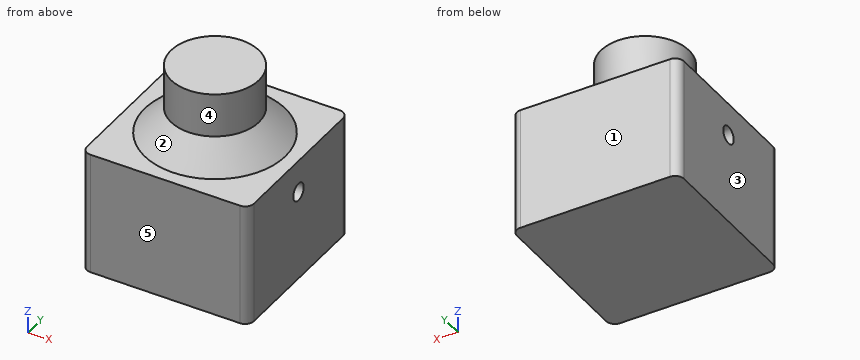
```python
from build123d import *

# Parameters (mm, degrees)
SKETCH1_W           = 19
SKETCH1_H           = 19
BOSS_EXTRUDE1_DEPTH = 14
FILLET1_R           = 1
SKETCH2_R           = 5
BOSS_EXTRUDE2_DEPTH = 8
CHAMFER1_SIZE       = 3
SKETCH3_R           = 1
CUT_EXTRUDE1_DEPTH  = 5
CUT_EXTRUDE2_START  = -5
SKETCH4_R           = 1
CUT_EXTRUDE2_DEPTH  = 5


with BuildPart() as part:
    # Sketch1 → Boss-Extrude1 (new body)
    with BuildSketch(Plane.XY):
        with Locations((66.227433771, 51.961607523)):
            Rectangle(SKETCH1_W, SKETCH1_H)
    extrude(amount=BOSS_EXTRUDE1_DEPTH)

    # Fillet1
    fillet1_edges = [part.edges().sort_by_distance(p)[0] for p in [
        (56.727433771, 61.461607523, 7),
        (75.727433771, 61.461607523, 7),
        (75.727433771, 42.461607523, 7),
        (56.727433771, 42.461607523, 7),
    ]]
    fillet(fillet1_edges, radius=FILLET1_R)

    # Sketch2 → Boss-Extrude2 (add)
    with BuildSketch(Plane.XY.offset(14)):
        with Locations((66.227433771, 51.961607523)):
            Circle(SKETCH2_R)
    extrude(amount=BOSS_EXTRUDE2_DEPTH)

    # Chamfer1
    chamfer1_edges = [part.edges().sort_by_distance(p)[0] for p in [
        (61.227433771, 51.961607523, 14),
    ]]
    chamfer(chamfer1_edges, length=CHAMFER1_SIZE)

    # Sketch3 → Cut-Extrude1 (cut)
    with BuildSketch(Plane.ZY.offset(-56.727433771)):
        with Locations(Location((10.3, 51.961607523, 0), (0, 0, 270))):
            Circle(SKETCH3_R)
    extrude(amount=-CUT_EXTRUDE1_DEPTH, mode=Mode.SUBTRACT)

    # Sketch4 → Cut-Extrude2 (cut)
    with BuildSketch(Plane(origin=(75.727433771, 0, 0), x_dir=(0, 0, -1), z_dir=(1, 0, 0)).offset(CUT_EXTRUDE2_START)):
        with Locations(Location((-10.3, 51.961607523, 0), (0, 0, 270))):
            Circle(SKETCH4_R)
    extrude(amount=CUT_EXTRUDE2_DEPTH, mode=Mode.SUBTRACT)


solid = part.part
```
Here's how the part is built. I have some questions about the finished solid (model axes, mm). Face numbers are marked on the shaded views. A direction names the side the tool comes from. Coordinates: 2 decimals unless noted, no trailing zeros. Loops run counter-clockwise (first coordinate to the right, second up) from the corner with the lowest first, then second, coordinate; pieces in that order, holes last. Notation, with made-up numbers: (-34.75, 71.25) -> (2.25, 71.25) arc R28 ccw to (2.25, 106.25) -> close; hole circle Ø5 at (51.25, 22). An arc over 180 degrees is marked (long way). Return JSON: item names as keys, results as strings.
1) Thinking about a two-plate mould opening in X: for the marked faces 1, 2 and 3, which applies, +X half, -X half, draft (parallel to the pull), parting line (faces both ways), or undercut?
Results below:
{"face 1": "draft", "face 2": "parting line", "face 3": "-X half"}
2) Will these pins go through, and if not, where does the flat tip stop? pin 1 (5 mm diameter, centred on y = 44.5, z = 14.5, fed in from +X); pin 2 (1 mm diameter, centred on y = 52, z = 10, fed in from -X); pin 3 (1.2 mm diameter, centred on y = 51.96, z = 10.3, fed in from +X).
Results below:
{"pin 1": "x = 75.73", "pin 2": "x = 61.73", "pin 3": "x = 70.73"}
3) If we section it at A-A, the plane z = 10.3: Write out the boundary of the cut face in (x, y).
Results below:
{"outline": "(56.73, 43.46) arc R1 ccw to (57.73, 42.46) -> (74.73, 42.46) arc R1 ccw to (75.73, 43.46) -> (75.73, 50.96) -> (70.73, 50.96) -> (70.73, 52.96) -> (75.73, 52.96) -> (75.73, 60.46) arc R1 ccw to (74.73, 61.46) -> (57.73, 61.46) arc R1 ccw to (56.73, 60.46) -> (56.73, 52.96) -> (61.73, 52.96) -> (61.73, 50.96) -> (56.73, 50.96) -> close"}
4) I need wall thicknesses on line 1 (Y direction, x = 74.6, z = 10.3); line 2 (Z direction, x = 59.5, y = 46.5); line 3 (Y direction, x = 59, z = 10). Which ranges of each line are inside material? Lowest first, please. Write a range as from..to.
Results below:
{"line 1": "42.46..50.96, 52.96..61.46", "line 2": "0..14", "line 3": "42.46..51.01, 52.92..61.46"}
5) For the marked faces 4 and 5, which set-ups out of +Z, -Z, +X, -X, +Y, -Y let a thin tool reach every point of the face, with its end or its side?
Results below:
{"face 4": "+Z", "face 5": "+Z, -Z, +X, -X, -Y"}
6) If we section it at B-B, the plane z = 16.25: Write out the boundary of the cut face in (x, y), then the cut area to 3 significant figures.
Results below:
{"outline": "circle Ø11.5 at (66.23, 51.96)", "area": "104 mm²"}
